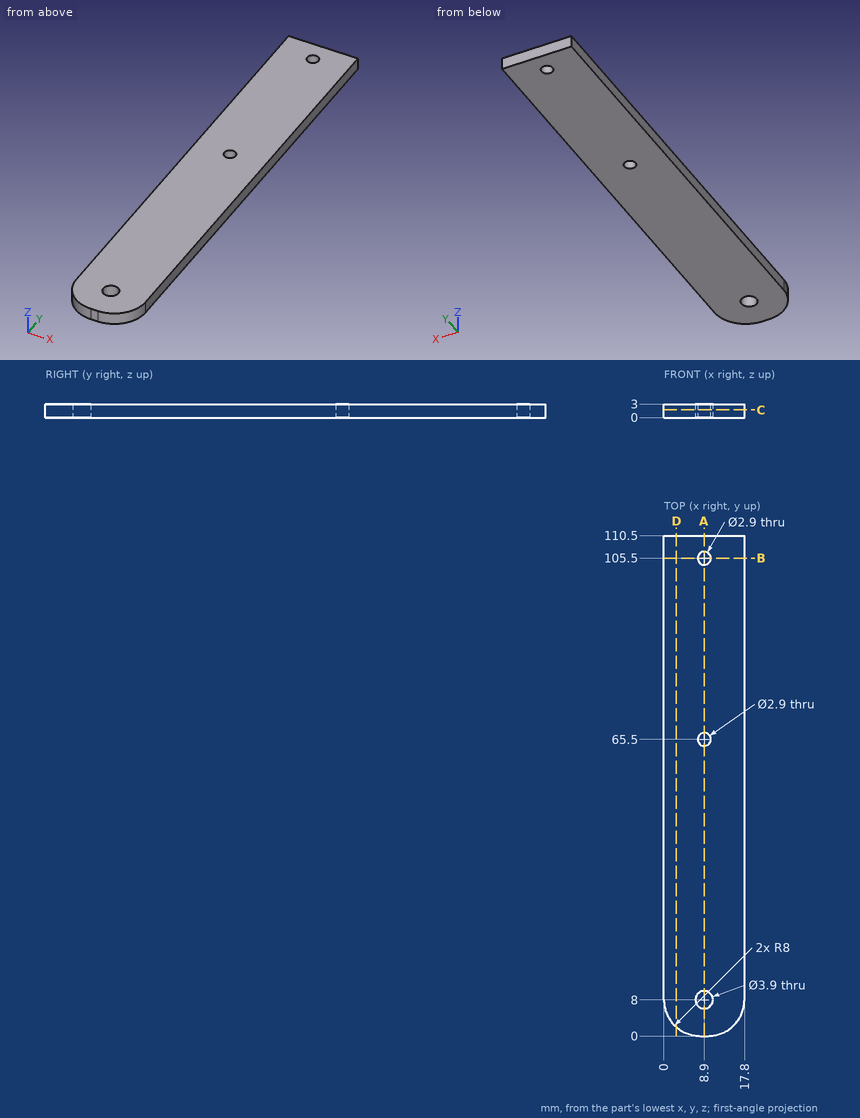
Check sheet for the drawn part. Datum: minimum x, y, z corner. Units: mm. Coordinates: 2 decimals unless noted, no trailing zeros. Order: outer loops, then holes, each group sorted by start corner. A loop starts at its lowest first (then second) coordinate and runs counter-clockwise, first axis right, second up. Notation, with made-up numbers: M 30,79.25 L 35,79.25 A17 cw 35,104.25 Z; hole C 20,-3 d11. An arc over 180 degrees is marked long. One line per question, with ' | ' between items. Start each with the question number.
Item 1: Gauge pin test, flat ends, axial feed: pin 1 (4.5 mm diameter, centred on x = 8.9, y = 8, fed in from +Z); pin 2 (2.5 mm diameter, centred on x = 8.9, y = 65.5, fed in from -Z). Record the tip position at first contact, or that the pin passes through.
Item 2: Cross-section at A-A on x = 8.9. Enter the section's corners in (y, z).
Item 3: Cross-section at C-C on z = 1.7. Enter the section's corners in (x, y), then the cut area to 3 significant figures.
Item 4: Cross-section at D-D on x = 2.75. Enter the section's corners in (y, z), then the cut area to 3 significant figures.
Item 5: Material ranges on L1, parallel to Y at x = 8.9, z = 1.25; L2, parallel to Y at x = 8.25, z = 1.65; L3, parallel to X at y = 65.5, z = 2.3, recorded low to high. Write a range as [from, to].
Item 6: Cross-section at B-B on y = 105.5. Enter the section's corners in (x, z).
Findings:
1) pin 1: stops at z = 3 | pin 2: passes through
2) outline: M 0,0 L 6.05,0 L 6.05,3 L 0,3 Z; M 9.95,0 L 64.05,0 L 64.05,3 L 9.95,3 Z; M 66.95,0 L 104.05,0 L 104.05,3 L 66.95,3 Z; M 106.95,0 L 110.5,0 L 110.5,3 L 106.95,3 Z
3) outline: M 0,8 A8 ccw 8,0 L 9.8,0 A8 ccw 17.8,8 L 17.8,110.5 L 0,110.5 Z; hole C 8.9,8 d3.9; hole C 8.9,65.5 d2.9; hole C 8.9,105.5 d2.9 | area: 1,910 mm²
4) outline: M 1.96,0 L 110.5,0 L 110.5,3 L 1.96,3 Z | area: 326 mm²
5) L1: y = [0, 6.05], [9.95, 64.05], [66.95, 104.05], [106.95, 110.5] | L2: y = [0, 6.16], [9.84, 64.2], [66.8, 104.2], [106.8, 110.5] | L3: x = [0, 7.45], [10.35, 17.8]
6) outline: M 0,0 L 7.45,0 L 7.45,3 L 0,3 Z; M 10.35,0 L 17.8,0 L 17.8,3 L 10.35,3 Z
